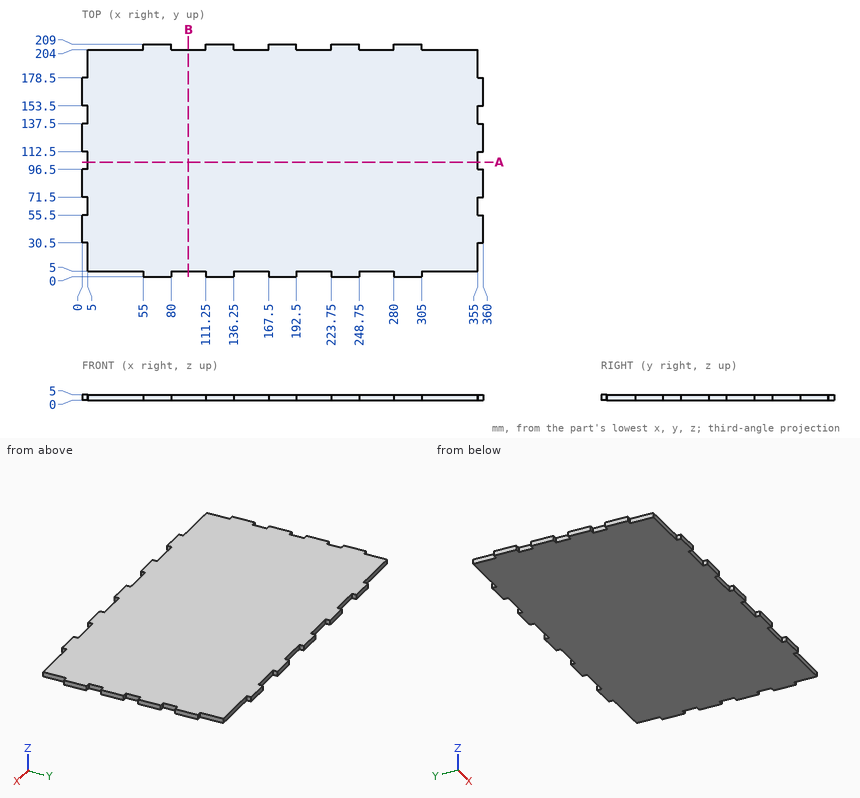
Geometry: see drawing. Coordinates: mm, zero at the bounding-box minimum. Coordinates: 2 decimals unless noted, no trailing zeros. Write each loop counter-clockwise with the first axis right and the second up, starting at its lowest first coordinate (ties: lowest second). Pieces come first, ordered by that corner, then holes. Notation, with made-up numbers: (47.5, -39.75) - (73.5, -39.75) arc R24 cw to (73.5, -29.75) - close; hole circle Ø7 at (23, 62.5). An arc over 180 degrees is marked (long way). Put each result on its own line as item: value. Start each with the question number.
1) Ray query, L1, parallel to X at y = 59.5, z = 2.2; L2, parallel to Y at x = 214, z = 2.75. Return the intervals inside material, ascending.
2) Contact query for flat-ended pins moving along their axis: pin 1 (2.5 mm diameter, centred on x = 204, z = 2, fed in from -Y); pin 2 (2.5 mm diameter, centred on y = 193, z = 2, fed in from -X); pin 3 (2.5 mm diameter, centred on y = 2.5, z = 1.5, fed in from +X). Output: stop coordinate, or through.
3) Cut plane A-A (y = 103). Return the cut outline in (x, z), plus the area to 3 significant figures.
4) Cut plane B-B (x = 95.5). Return the cut outline in (y, z).
Resolved:
1. L1: x = 5 to 355
1. L2: y = 5 to 204
2. pin 1: stops at y = 5
2. pin 2: stops at x = 5
2. pin 3: stops at x = 305
3. outline: (5, 0) - (355, 0) - (355, 5) - (5, 5) - close
3. area: 1,750 mm2
4. outline: (5, 0) - (204, 0) - (204, 5) - (5, 5) - close
